The model under review builds one solid part; all positions refer to its coordinate system, in mm. Round coordinates to 2 decimals unless told otherwise and drop trailing zeros. Loops run counter-clockwise (first coordinate to the right, second up) from the corner with the lowest first, then second, coordinate; pieces in that order, holes last. Notation, with made-up numbers: (47, 77.25) -> (100, 77.25) arc R11 cw to (100, 82.25) -> close; hole circle Ø5 at (72, 6). An arc over 180 degrees is marked (long way). Write each question's results on one line, items separated by ' | '. Start each with the question number.
Item 1: For L1, parallel to Y at x = 0, z = 37; L2, parallel to Z at x = -8, y = -3.5; L3, parallel to Y at x = -17, z = 41, list the stretches that pass through material, from the lowest coordinate up. Write a range as from..to.
Item 2: We need section C-C (z = 19). Give the boundary of the cut face in (x, y), and give its area (3 significant figures).
Item 3: Clearance check with flat-ended pins moving along their axes: pin 1 Ø6 at (x, z) = (34, 50) entering from -Y; pin 2 Ø1.5 at (x, z) = (8, 98) entering from -Y; pin 3 Ø10 at (y, z) = (13.5, 46.5) entering from +X. State where each tip first meets the part, or that it passes through.
Item 4: Mouldability with a two-part tool opening along Y and no side actions: class faces 1 (the flat face through (-1, 1, 0)), 2 (the cylindrical face through (-10, -43, 55)), 3 (the flat face through (-1, 1, 7.62)), 4 (the cylindrical face through (34.84, 10.97, 58.4)) as pulls with the +Y half, pulls with the -Y half, needs draft (parallel to the pull), parting line crosses it, or undercut.
Item 5: We need section A-A (y = 0). Give the boundary of the cut face in (x, z), and give its area (3 significant figures).
from build123d import *

# Parameters (mm, degrees)
F0_R     = 44.1474000208
F1_DEPTH = 114.3
F2_T     = -7.62
F3_R     = 3.6792614691


with BuildPart() as f1:
    # F0 (on Top) → F1 (new body)
    with BuildSketch(Plane.XY):
        Circle(F0_R)
    extrude(amount=F1_DEPTH)

    # F2
    f2_openings = [f1.faces().sort_by_distance(p)[0] for p in [
        (0, 0, 114.3),
    ]]
    offset(amount=F2_T, openings=f2_openings)

    # F3
    f3_edges = [f1.edges().sort_by_distance(p)[0] for p in [
        (-44.1474, 0, 114.3),
        (-36.5274, 0, 114.3),
    ]]
    fillet(f3_edges, radius=F3_R)


solid = f1.part
Here are the results:
1) L1: y = -44.15..-36.53, 36.53..44.15 | L2: z = 0..7.62 | L3: y = -40.74..-32.33, 32.33..40.74
2) outline: circle Ø88.29 at (0, 0); hole circle Ø73.05 at (0, 0) | area: 1,930 mm2
3) pin 1: stops at y = -31.43 | pin 2: stops at y = -43.55 | pin 3: stops at x = 43.32
4) face 1: needs draft | face 2: parting line crosses it | face 3: undercut | face 4: undercut
5) outline: (-44.15, 0) -> (44.15, 0) -> (44.15, 110.62) arc R3.68 ccw to (40.47, 114.3) -> (40.21, 114.3) arc R3.68 ccw to (36.53, 110.62) -> (36.53, 7.62) -> (-36.53, 7.62) -> (-36.53, 110.62) arc R3.68 ccw to (-40.21, 114.3) -> (-40.47, 114.3) arc R3.68 ccw to (-44.15, 110.62) -> close | area: 2,290 mm2
